The listing builds one solid part. Answer for the finished solid, in the listing's coordinates (mm). Give positions to 0.01 mm unless a question says otherwise; leave off trailing zeros. Loops run counter-clockwise (first coordinate to the right, second up) from the corner with the lowest first, then second, coordinate; pieces in that order, holes last.
Item 1: Section B-B, the plane y = 0.6 is taken. Give the vertices of the cut face in (x, z).
Item 2: Section A-A, the plane x = -4.25 is taken. Give the vertices of the cut face in (y, z), and give its area (3 significant figures).
Item 3: The mould has two halves that part along Z. Classify faces 1 (the face through (-10, 5, 47)), 2 (the face through (-8.726, 2.535, 32.243)), 3 (the face through (0.294, 2.535, 77.367)): pulls with the +Z half, pulls with the -Z half, needs draft (parallel to the pull), parting line crosses it, or undercut.
Item 4: Each of these flat-tipped pins is pushed along its axis until it touches: pin 1 Ø1 at (y, z) = (3, 39.5) entering from -X; pin 2 Ø1.5 at (x, y) = (-11, 3) entering from -Z; pin 3 Ø2 at (y, z) = (1, 66) entering from -X. Where does it stop, or does it pass through?
Item 5: Section C-C, the plane x = -8.75 is taken. Give the vertices of the cut face in (y, z).
Item 6: Section D-D, the plane z = 40 is taken. Give the vertices of the cut face in (x, y).
Item 7: Consider line 1 along Z through (x, y) = (-2.5, 0.7); line 2 along Z through (x, y) = (-7.5, 0.6); line 3 along X through (y, z) = (3.65, 45.5). Determine where each line is inside the solid, lowest interval first.
from build123d import *

# Parameters (mm, degrees)
EXTRUDE_2_DEPTH     = 5
SKETCH_4_R          = 1.65
CUT_EXTRUDE_1_DEPTH = 5
EXTRUDE_3_DEPTH     = 5
CUT_EXTRUDE_START   = -4.5
SKETCH_7_R          = 3
CUT_EXTRUDE_2_DEPTH = 3
CUT_EXTRUDE_3_DEPTH = 7.5
EXTRUDE_4_DEPTH     = 5
FILLET_1_R          = 5
FILLET_2_R          = 5
CUT_EXTRUDE_START_2 = -5
CUT_EXTRUDE_5_DEPTH = 5


with BuildPart() as part:
    # 草图3 → 凸台-拉伸2 (new body)
    with BuildSketch(Plane(origin=(0, 0, 0), x_dir=(1, 0, 0), z_dir=(0, 1, 0))):
        with BuildLine():
            Line((-3, -3.354101966), (-3, -7.416198487))
            Line((-3, -7.416198487), (-3, -43.854101966))
            Line((-3, -43.854101966), (3, -43.854101966))
            Line((3, -43.854101966), (3, -10.583005244))
            Line((3, -10.583005244), (3, -7.416198487))
            Line((3, -7.416198487), (3, -3.354101966))
            ThreePointArc((3, -3.354101966), (0, 4.5), (-3, -3.354101966))
        make_face()
    extrude(amount=EXTRUDE_2_DEPTH)

    # 草图4 → 切除-拉伸1 (cut)
    with BuildSketch(Plane(origin=(0, 5, 0), x_dir=(1, 0, 0), z_dir=(0, 1, 0))):
        with Locations(Location((0, 0, 0), (0, 0, 270))):
            Circle(SKETCH_4_R)
    extrude(amount=-CUT_EXTRUDE_1_DEPTH, mode=Mode.SUBTRACT)

    # 草图6 → 凸台-拉伸3 (add)
    with BuildSketch(Plane(origin=(0, 5, 0), x_dir=(1, 0, 0), z_dir=(0, 1, 0))):
        with BuildLine():
            Line((3, -33.74604712), (-3, -33.74604712))
            ThreePointArc((-3, -33.74604712), (-16.46902092, -57.986607816), (0.722500961, -79.745993902))
            Line((0.722500961, -79.745993902), (1.949520222, -77.620734201))
            ThreePointArc((1.949520222, -77.620734201), (-10.543317179, -55.371702353), (3, -33.74604712))
        make_face()
    extrude(amount=-EXTRUDE_3_DEPTH)

    # 草图7 → 切除-拉伸2 (cut)
    with BuildSketch(Plane(origin=(0, 5, 0), x_dir=(1, 0, 0), z_dir=(0, 1, 0)).offset(CUT_EXTRUDE_START)):
        with Locations(Location((0, 0, 0), (0, 0, 270))):
            Circle(SKETCH_7_R)
    extrude(amount=-CUT_EXTRUDE_2_DEPTH, mode=Mode.SUBTRACT)

    # 草图8 → 切除-拉伸3 (cut)
    with BuildSketch(Plane(origin=(0, 5, 0), x_dir=(1, 0, 0), z_dir=(0, 1, 0))):
        with BuildLine():
            Line((-3, -38.067187498), (-3, -43.854101966))
            Line((-3, -43.854101966), (3, -43.854101966))
            Line((3, -43.854101966), (3, -33.74604712))
            ThreePointArc((3, -33.74604712), (-0.160637142, -35.683569047), (-3, -38.067187498))
        make_face()
    extrude(amount=-CUT_EXTRUDE_3_DEPTH, mode=Mode.SUBTRACT)

    # 草图9 → 凸台-拉伸4 (add)
    with BuildSketch(Plane(origin=(0, 5, 0), x_dir=(1, 0, 0), z_dir=(0, 1, 0))):
        with BuildLine():
            Line((-3, -18.550074543), (-14.614967684, -46.324924269))
            ThreePointArc((-14.614967684, -46.324924269), (-9.917875534, -39.010182445), (-3, -33.74604712))
            Line((-3, -33.74604712), (-3, -18.550074543))
        make_face()
    extrude(amount=-EXTRUDE_4_DEPTH)

    # 圆角1
    fillet_1_edges = [part.edges().sort_by_distance(p)[0] for p in [
        (3, 2.5, 33.74604712),
    ]]
    fillet(fillet_1_edges, radius=FILLET_1_R)

    # 圆角2
    # the kernel refuses this fillet: 5 mm, written as the material it takes off along each edge
    with BuildSketch(Plane(origin=(1.949520222, 14.371610933, 77.620734201), x_dir=(-0.8261015944022844, 0, -0.5635212114250925), z_dir=(0, -1, 0))) as fillet_2_piece_1:
        with BuildLine():
            CenterArc((4.123508811, -4.985927863), FILLET_2_R, 94.299664485, 55.185648669)
            Line((-0.183986354, -2.447131808), (-0.270136257, -2.396355887))
            ThreePointArc((-0.270136257, -2.396355887), (-0.191711734, -1.216068615), (-0.099718557, 0.007497289))
            Line((-0.099718557, 0.007497289), (0.007497289, 0.099718557))
            ThreePointArc((0.007497289, 0.099718557), (1.874322187, 0.029639314), (3.741147084, 0.099718557))
            Line((3.741147084, 0.099718557), (3.748644373, 0))
        make_face()
    extrude(amount=23.743221866, mode=Mode.SUBTRACT)

    # 草图10 → 切除-拉伸5 (cut)
    with BuildSketch(Plane(origin=(0, 5, 0), x_dir=(1, 0, 0), z_dir=(0, 1, 0)).offset(CUT_EXTRUDE_START_2)):
        with BuildLine():
            Line((-3, -18.550074543), (3, -18.550074543))
            Line((3, -18.550074543), (3, -3.354101966))
            ThreePointArc((3, -3.354101966), (0, 4.5), (-3, -3.354101966))
            Line((-3, -3.354101966), (-3, -18.550074543))
        make_face()
    extrude(amount=CUT_EXTRUDE_5_DEPTH, mode=Mode.SUBTRACT)


solid = part.part
Worked answers:
1. outline: (-14.61, 46.32) - (-3, 18.55) - (3, 18.55) - (3, 30.88) arc R5 ccw to (0.74, 35.06) arc R25 cw to (-1.15, 75.51) arc R5 ccw to (0.72, 79.75) arc R25 ccw to start
2. outline: (0, 21.54) - (5, 21.54) - (5, 39.38) - (0, 39.38) - close; (0, 72.56) - (5, 72.56) - (5, 77.5) - (0, 77.5) - close
2. area: 114 mm2
3. face 1: needs draft
3. face 2: pulls with the -Z half
3. face 3: undercut
4. pin 1: stops at x = -11.97
4. pin 2: stops at z = 35.89
4. pin 3: stops at x = -14.86
5. outline: (0, 32.3) - (5, 32.3) - (5, 46.65) - (0, 46.65) - close; (0, 65.29) - (5, 65.29) - (5, 74.11) - (0, 74.11) - close
6. outline: (-11.97, 0) - (-4.78, 0) - (-4.78, 5) - (-11.97, 5) - close
7. line 1: z = 18.55 to 37.59, 74.35 to 78.44
7. line 2: z = 29.31 to 44, 67.94 to 75.22
7. line 3: x = -14.27 to -8.25
